Geometry: see drawing. Coordinates: mm, zero at the bounding-box minimum. A direction names the side the tool comes from. Give positions to 0.01 mm unless a question says otherwise; leave off trailing zeros. Write each loop counter-clockwise with the first axis right and the second up, starting at its lowest first coordinate (ties: lowest second). Pieces come first, ordered by that corner, then holes. Notation, with made-up numbers: M -30,77.25 L 18,77.25 A3 ccw 18,81.25 Z; hole C 16.25,65 d5. An arc over 180 degrees is marked long. Use one line per item in the form item = value. Start each with the question number.
Item 1: Material intervals for line 1 along Z through (x, y) = (7.25, 23) (1 decimal); line 2 along Y through (x, z) = (10.5, 17.5); line 3 along Z through (x, y) = (15.25, 9.5) (1 decimal), sorted ascending. Write a range as from..to.
Item 2: Access query for the marked faces 1 and 2. Directions: +Z, -Z, +X, -X, +Y, -Y. A direction counts if a zero-diameter tool reaches every point of the face in a straight line with its end or side. Return the directions, or none.
Item 3: Section query A-A on x = 9.25. Return loops of the section in (y, z), then the cut area to 3 significant figures.
Item 4: Pull-direction query (Z, two-part tool) for the marked faces 3, 4 and 5; classes: released by +Z, released by -Z, zero draft, split by the parting line, or undercut.
Item 5: Section query B-B on x = 4. Return loops of the section in (y, z) (1 decimal), then the cut area to 3 significant figures.
Item 6: Contact query for flat-ended pins moving along their axis: P1, Ø5, axis at x = 8.5, y = 4.5, coming from the +Z side; P2, Ø6, axis at x = 10, y = 24, coming from the +Z side; P3, Ø1, axis at x = 6.5, y = 28.5, coming from the +Z side. Output: stop coordinate, or through.
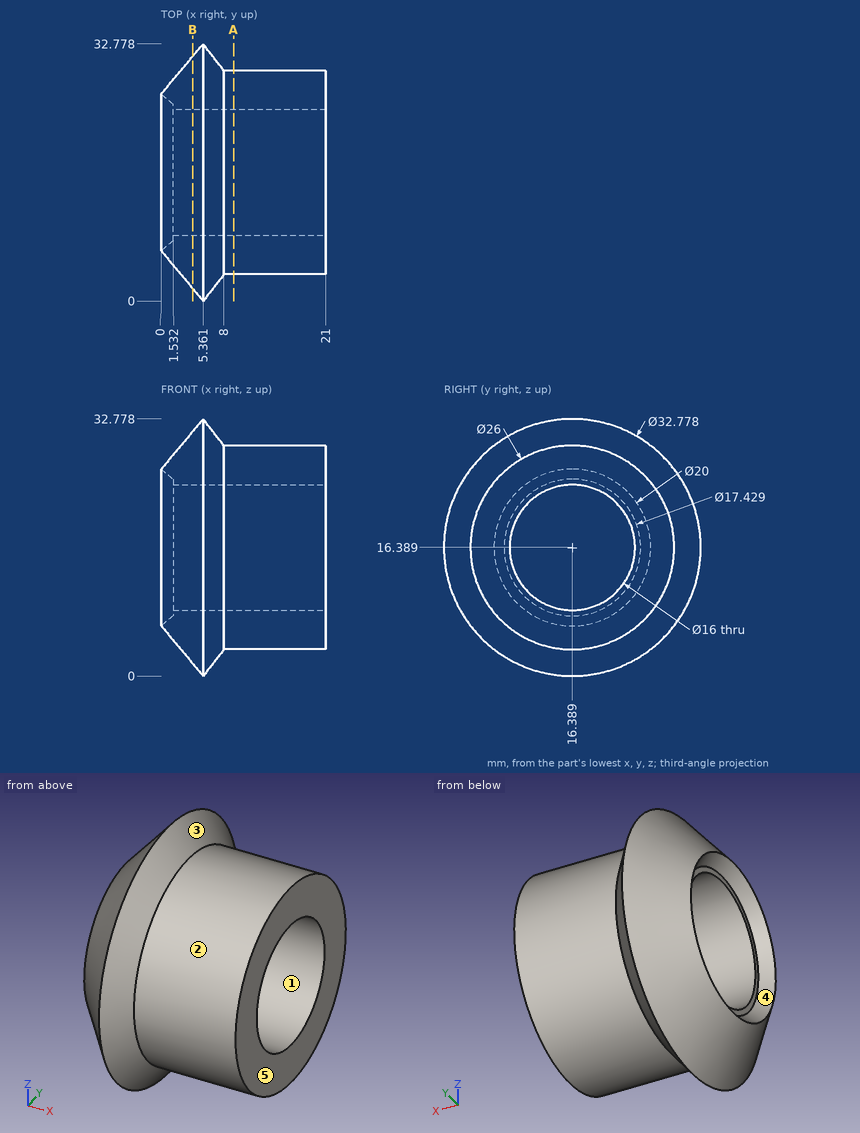
Answer sheet:
q1.line_1 = 4.1..11.9, 20.9..28.7
q1.line_2 = 3.44..8.47, 24.31..29.34
q1.line_3 = 5.4..12.3, 20.5..27.4
q2.face_1 = +X, -X
q2.face_2 = +X
q3.outline = C 16.39,16.39 d26; hole C 16.39,16.39 d16
q3.area = 330 mm2
q4.face_3 = split by the parting line
q4.face_4 = undercut
q4.face_5 = zero draft
q5.outline = C 16.4,16.4 d29.5; hole C 16.4,16.4 d16
q5.area = 484 mm2
q6.P1 = 27.16
q6.P2 = 28.8
q6.P3 = 26.34
